Check sheet for the drawn part. Datum: minimum x, y, z corner. Units: mm. A direction names the side the tool comes from. Coordinates: 2 decimals unless noted, no trailing zeros. Write each loop counter-clockwise with the first axis right and the second up, starting at its lowest first coordinate (ties: lowest second). Pieces come first, ordered by that corner, then holes. Notation, with made-up numbers: M -34.5,30 L -19.5,30 A18 cw -19.5,34 Z; hole C 34,40.25 d1. An arc over 180 degrees is marked long. Answer as CSV lines item,"result".
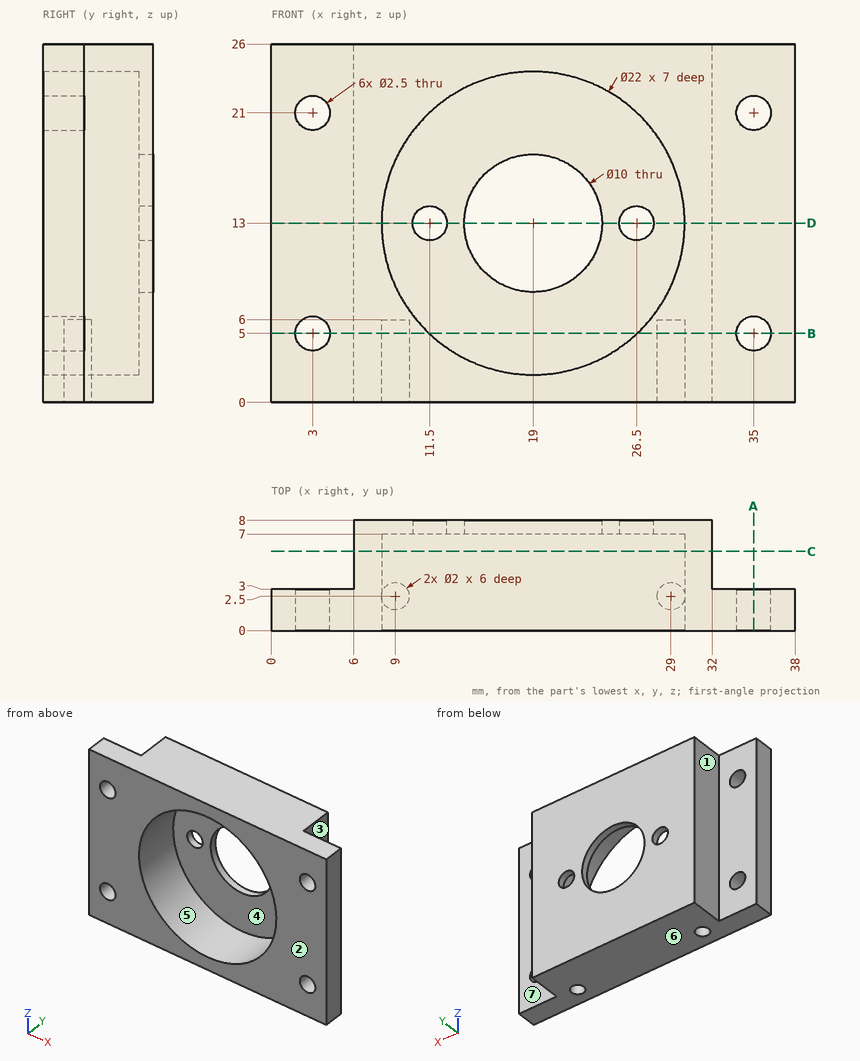
1) Section check B-B, the plane z = 5. Record the boundary of the cut face in (x, y), plus the area to 3 significant figures.
Answer key:
outline,"M 0,0 L 1.75,0 L 1.75,3 L 0,3 Z; M 4.25,0 L 11.45,0 L 11.45,7 L 26.55,7 L 26.55,0 L 33.75,0 L 33.75,3 L 32,3 L 32,8 L 6,8 L 6,3 L 4.25,3 Z; M 36.25,0 L 38,0 L 38,3 L 36.25,3 Z; hole C 9,2.5 d2; hole C 29,2.5 d2"
area,"117 mm2"
2) Tool access check on the marked faces 1, 2 and 3. Record the directions out of +Z, -Z, +X, -X, +Y, -Y that give a thin tool (end or side, any length) a straight path to the whole face; none if there is none.
Answer key:
face 1,"+Z, -Z, -X, +Y"
face 2,"+Z, -Z, +X, -X, -Y"
face 3,"+Z, -Z, +X, +Y"
3) Section check C-C, the plane y = 5.75. Record the boundary of the cut face in (x, z), plus the area to 3 significant figures.
Answer key:
outline,"M 6,0 L 32,0 L 32,26 L 6,26 Z; hole C 19,13 d22"
area,"296 mm2"
4) Section check D-D, the plane z = 13. Record the boundary of the cut face in (x, y), plus the area to 3 significant figures.
Answer key:
outline,"M 0,0 L 8,0 L 8,7 L 10.25,7 L 10.25,8 L 6,8 L 6,3 L 0,3 Z; M 12.75,7 L 14,7 L 14,8 L 12.75,8 Z; M 24,7 L 25.25,7 L 25.25,8 L 24,8 Z; M 27.75,7 L 30,7 L 30,0 L 38,0 L 38,3 L 32,3 L 32,8 L 27.75,8 Z"
area,"75.0 mm2"
5) Thickness scan on line 1 along Z through (x, y) = (3, 1); line 2 along Z through (x, y) = (11.5, 7.7); line 3 along X through (y, z) = (4, 23). Record the ranges inside material, lowest first.
Answer key:
line 1,"z = 0 to 3.75, 6.25 to 19.75, 22.25 to 26"
line 2,"z = 0 to 11.75, 14.25 to 26"
line 3,"x = 6 to 14.42, 23.58 to 32"
6) Depth check by flat-ended pin: P1, Ø6.5, axis at x = 14, z = 17, coming from the -Y side; P2, Ø1.5, axis at y = 5, z = 17.5, coming from the +X side; P3, Ø4, axis at x = 35, z = 5, coming from the +Y side; P4, Ø2, axis at x = 3, z = 21, coming from the +Y side. Enter the tip coordinate at first touch or a pass-through.
Answer key:
P1,"stops at y = 7"
P2,"stops at x = 32"
P3,"stops at y = 3"
P4,"passes through"
7) Section check A-A, the plane x = 35. Record the boundary of the cut face in (y, z).
Answer key:
outline,"M 0,0 L 3,0 L 3,3.75 L 0,3.75 Z; M 0,6.25 L 3,6.25 L 3,19.75 L 0,19.75 Z; M 0,22.25 L 3,22.25 L 3,26 L 0,26 Z"
8) Mould release check, pull along Z, two halves, no side actions. Record for the marked faces 4, 5, 6 and 7: pulls with the +Z half, pulls with the -Z half, needs draft (parallel to the pull), parting line crosses it, or undercut.
Answer key:
face 4,"undercut"
face 5,"undercut"
face 6,"pulls with the -Z half"
face 7,"needs draft"
